Autodesk Fusion 360 part; units mm, degrees
sketch "Sketch1" plane through (0, 0, 0) normal (0, 0, 1) x (1, 0, 0)
  line L0 (-1.1, 1.1) -> (-1.1, 5.1)
  arc A0 (1.1, 5.1) -> (-1.1, 5.1) centre (0, 5.1) ccw
  line L1 (1.1, 5.1) -> (1.1, 1.1)
  line L2 (-1.1, 5.1) -> (1.1, 5.1) construction
  line L3 (1.1, 1.1) -> (-1.1, 1.1) construction
  line L4 (-1.1, 1.1) -> (-1.1, -1.1) construction
  line L5 (-1.1, -1.1) -> (1.1, -1.1) construction
  line L6 (1.1, -1.1) -> (1.1, 1.1) construction
  line L7 (1.1, 1.1) -> (-1.1, -1.1) construction
  line L8 (-1.1, 1.1) -> (1.1, -1.1) construction
  line L9 (-1.1, -1.1) -> (-5.1, -1.1)
  arc A1 (-5.1, 1.1) -> (-5.1, -1.1) centre (-5.1, 0) ccw
  line L10 (-5.1, 1.1) -> (-1.1, 1.1)
  line L11 (1.1, -1.1) -> (1.1, -5.1)
  arc A2 (-1.1, -5.1) -> (1.1, -5.1) centre (0, -5.1) ccw
  line L12 (-1.1, -5.1) -> (-1.1, -1.1)
  line L13 (1.1, 1.1) -> (5.1, 1.1)
  arc A3 (5.1, -1.1) -> (5.1, 1.1) centre (5.1, 0) ccw
  line L14 (5.1, -1.1) -> (1.1, -1.1)
  line L15 (7.1, 7.1) -> (-7.1, 7.1)
  line L16 (-7.1, 7.1) -> (-7.1, -7.1)
  line L17 (-7.1, -7.1) -> (7.1, -7.1)
  line L18 (7.1, -7.1) -> (7.1, 7.1)
  line L19 (7.1, 7.1) -> (-7.1, -7.1) construction
  line L20 (-7.1, 7.1) -> (7.1, -7.1) construction
  dimension "d2" = 2.2
  dimension "d3" = 2.2
  dimension "d4" = 2.2
  dimension "d5" = 4
  dimension "d7" = 360
  dimension "d37" = 2
extrude "Extrude1" add sketch "Sketch1" along normal blind 3
sketch "Sketch2" plane through (0, 0, 0) normal (0, 0, 1) x (1, 0, 0)
  line L0 (-33.9, 6.35) -> (-21.2, 6.35) construction
  line L1 (-21.2, 6.35) -> (-21.2, -6.35) construction
  line L2 (-21.2, -6.35) -> (-33.9, -6.35) construction
  line L3 (-33.9, -6.35) -> (-33.9, 6.35) construction
  line L4 (21.2, 6.35) -> (33.9, 6.35) construction
  line L5 (33.9, 6.35) -> (33.9, -6.35) construction
  line L6 (33.9, -6.35) -> (21.2, -6.35) construction
  line L7 (21.2, -6.35) -> (21.2, 6.35) construction
  line L8 (-21.2, 0) -> (21.2, 0) construction
  line L9 (-21.1, -6.45) -> (-34, -6.45)
  line L10 (-34, -6.45) -> (-34, 6.45)
  line L11 (-34, 6.45) -> (-21.1, 6.45)
  line L12 (-21.1, 6.45) -> (-21.1, -6.45)
  line L13 (-18.6, -8.95) -> (-36.5, -8.95)
  line L14 (-36.5, -8.95) -> (-36.5, 8.95)
  line L15 (-36.5, 8.95) -> (-18.6, 8.95)
  line L16 (-18.6, 8.95) -> (-18.6, -8.95)
  line L17 (0, 2.5) -> (0, 20)
  line L18 (34, -6.45) -> (34, 6.45)
  line L19 (34, 6.45) -> (21.1, 6.45)
  line L20 (21.1, 6.45) -> (21.1, -6.45)
  line L21 (21.1, -6.45) -> (34, -6.45)
  line L22 (36.5, -8.95) -> (36.5, 8.95)
  line L23 (36.5, 8.95) -> (18.6, 8.95)
  line L24 (18.6, -8.95) -> (36.5, -8.95)
  line L25 (18.6, 8.95) -> (18.6, -8.95)
  line L26 (-18.6, -2.6) -> (-18.6, -8.95)
  line L27 (-18.6, 8.95) -> (18.6, 8.95)
  line L28 (18.6, -8.95) -> (-18.6, -8.95)
  line L29 (-7.1, 7.1) -> (-7.1, -7.1)
  line L30 (-7.1, -7.1) -> (7.1, -7.1)
  line L31 (7.1, -7.1) -> (7.1, 7.1)
  line L32 (7.1, 7.1) -> (-7.1, 7.1)
  dimension "d18" = 12.7
  dimension "d19" = 12.7
  dimension "d20" = 42.4
  dimension "d23" = -2.5
extrude "Extrude2" add sketch "Sketch2" along normal blind 3
extrude "Extrude3" add sketch "Sketch2" against normal blind 19 contours L13 L14 L15 L16 L26 | L22 L23 L24 L25
fillet "Fillet1" radius 12 2 edges at (-18.6, 0, 0) (18.6, 0, 0)
sketch "Sketch3" plane through (0, 8.95, 0) normal (0, 1, 0) x (-1, 0, 0)
  line L0 (36.5, -19) -> (36.5, 3)
  line L1 (36.5, 3) -> (-36.5, 3)
  line L2 (18.6, -12) -> (18.6, -19)
  line L3 (-36.5, -19) -> (-18.6, -19)
  circle A0 centre (-27.55, -12.6) radius 2.075
  circle A1 centre (-27.55, -2.6) radius 2.075
  line L4 (-27.55, -19) -> (-27.55, 3) construction
  line L5 (-36.5, 3) -> (-36.5, -19)
  line L6 (-18.6, -19) -> (-18.6, -12)
  line L7 (18.6, -19) -> (36.5, -19)
  line L8 (0, 1.75) -> (0, 22.5)
  circle A2 centre (27.55, -12.6) radius 2.075
  circle A3 centre (27.55, -2.6) radius 2.075
  dimension "d32" = 4.15
  dimension "d33" = 10
  dimension "d34" = 5.6
extrude "Extrude4" cut sketch "Sketch3" against normal blind 17.9
sketch "Sketch4" plane through (0, 0, 3) normal (0, 0, 1) x (1, 0, 0)
  line L0 (36.5, -8.95) -> (36.5, 8.95)
  line L1 (36.5, 8.95) -> (-36.5, 8.95)
  line L2 (-36.5, 8.95) -> (-36.5, -8.95)
  line L3 (-36.5, -8.95) -> (36.5, -8.95)
  line L4 (-34, 6.45) -> (-21.1, 6.45)
  line L5 (-21.1, 6.45) -> (-21.1, -6.45)
  line L6 (-21.1, -6.45) -> (-34, -6.45)
  line L7 (-34, -6.45) -> (-34, 6.45)
  line L8 (34, -6.45) -> (21.1, -6.45)
  line L9 (21.1, -6.45) -> (21.1, 6.45)
  line L10 (21.1, 6.45) -> (34, 6.45)
  line L11 (34, 6.45) -> (34, -6.45)
  arc A0 (1.1, 5.1) -> (-1.1, 5.1) centre (0, 5.1) ccw
  line L12 (1.1, 5.1) -> (1.1, 1.1)
  line L13 (1.1, 1.1) -> (5.1, 1.1)
  arc A1 (5.1, -1.1) -> (5.1, 1.1) centre (5.1, 0) ccw
  line L14 (5.1, -1.1) -> (1.1, -1.1)
  line L15 (1.1, -1.1) -> (1.1, -5.1)
  arc A2 (-1.1, -5.1) -> (1.1, -5.1) centre (0, -5.1) ccw
  line L16 (-1.1, -5.1) -> (-1.1, -1.1)
  line L17 (-1.1, -1.1) -> (-5.1, -1.1)
  arc A3 (-5.1, 1.1) -> (-5.1, -1.1) centre (-5.1, 0) ccw
  line L18 (-5.1, 1.1) -> (-1.1, 1.1)
  line L19 (-1.1, 1.1) -> (-1.1, 5.1)
  line L20 (-21.1, 6.45) -> (-21.1, -6.45)
  line L21 (21.1, -6.45) -> (21.1, 6.45)
  line L22 (-21.1, 0) -> (21.1, 0) construction
  circle A4 centre (-14.1, 0) radius 2.075
  line L23 (0, 2.5) -> (0, 20)
  circle A5 centre (14.1, 0) radius 2.075
  dimension "d38" = 7
  dimension "d39" = 4.15
extrude "Extrude5" cut sketch "Sketch4" against normal blind 22 contours A4 | A5
ref_plane "WorkPlane1" through (0, 0, -6) normal (0, 0, -1) x (-1, 0, 0)
sketch "Sketch5" plane through (0, 0, -6) normal (0, 0, -1) x (-1, 0, 0)
  line L0 (-21.1, 6.45) -> (-21.1, -6.45)
  line L1 (21.1, -6.45) -> (21.1, 6.45)
  line L2 (-21.1, 0) -> (21.1, 0) construction
  circle A0 centre (-14.1, 0) radius 4.5
  line L3 (0, 1.75) -> (0, 22.5)
  circle A1 centre (14.1, 0) radius 4.5
  line L4 (-17.7, 2.7) -> (-17.7, -2.7)
  line L5 (17.7, 2.7) -> (17.7, -2.7)
  dimension "d43" = 9
  dimension "d44" = 7
  dimension "d49" = 3.6
extrude "Extrude6" cut sketch "Sketch5" along normal blind -6 and the other way blind -45.366 contours A0 L4 | A1 L5 picked at (-15.387, 1.0056) picked at (17.8896, 0.5649)
equation "mounting_size = 2.2 mm"
equation "d2 = mounting_size"
equation "d3 = mounting_size"
equation "d4 = mounting_size"
equation "tolerance_bar = 0.1 mm"
equation "d30 = 13 mm - ( 4 / 4 ) * 1 mm"
equation "tolerance_hole = 0.15 mm"
equation "d32 = 4 mm + tolerance_hole"
equation "d39 = 4 mm + tolerance_hole"
equation "d49 = ( 7 / 2 ) * 1 mm + 0.1 mm"
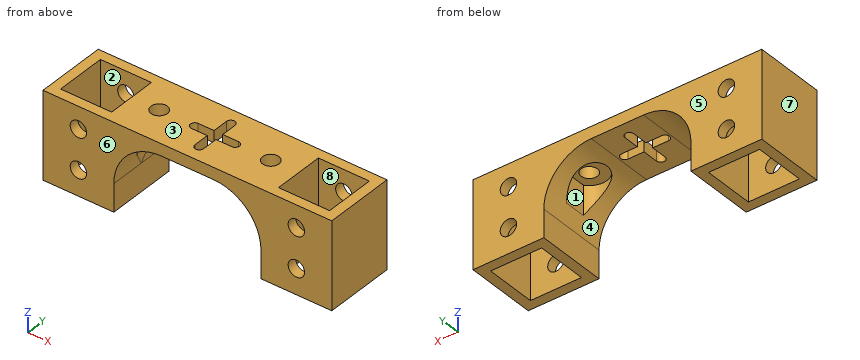
CAD build for the part. Positions are in the model's coordinates, mm. Face numbers are marked on the shaded views. A direction names the side the tool comes from. Round coordinates to 2 decimals unless told otherwise and drop trailing zeros. Write each loop counter-clockwise with the first axis right and the second up, starting at its lowest first coordinate (ties: lowest second). Pieces come first, ordered by that corner, then holes. Notation, with made-up numbers: (47, -29.5) - (71, -29.5) arc R17 ccw to (71, -9.5) - close; hole circle Ø3 at (85.25, 8). An arc over 180 degrees is marked (long way). Return JSON: item names as keys, results as strings. Group by question number.
Item 1: Band-saw the part on D-D on y = -7.5. List the corners of the cut face in (x, z) (3 decimals).
Item 2: 3-axis set-ups, long thin cutter, end or side, ignore diameter. For the marked faces 1, 2, 3, 4 and 5: which of +Z, -Z, +X, -X, +Y, -Y reach the whole face in a straight line?
Item 3: Band-saw the part on C-C on x = -27.55. List the corners of the cut face in (y, z) (3 decimals), plus the area to 3 significant figures.
Item 4: Band-saw the part on A-A on x = 3. List the corners of the cut face in (y, z).
Item 5: Band-saw the part on B-B on z = 1.5. List the corners of the cut face in (x, y) (3 decimals), plus the area to 3 significant figures.
Item 6: Probe probe 1 along X at (y, z) = (5.5, -13.25); probe 2 along X at (y, z) = (0, -4) (3 decimals); probe 3 along Y at (x, z) = (31.5, 0.5). List the from-to ranges inside material, lowest first.
Item 7: Flat gauge pins, fed straight in: pin 1 Ø0.7 at (x, y) = (-18, -0.5) entering from -Z; pin 2 Ø6.5 at (x, z) = (-27.55, -2.6) entering from -Y; pin 3 Ø3.5 at (x, z) = (27.55, -12.6) entering from -Y; pin 4 Ø10.5 at (x, y) = (-1, -4.5) entering from -Z. Where does each tip first touch, or does it go through?
Item 8: Mould opens along Y. For the marked faces 6, 7 and 8 say: +Y half, -Y half, draft (parallel to the pull), parting line (faces both ways), or undercut.
Resolved:
{
 "1": {"outline": "(-36.5, -19) - (-18.6, -19) - (-18.6, -12) arc R12 cw to (-6.6, 0) - (6.6, 0) arc R12 cw to (18.6, -12) - (18.6, -19) - (36.5, -19) - (36.5, 3) - (-36.5, 3) - close; hole circle Ø4.15 at (-27.55, -12.6); hole circle Ø4.15 at (-27.55, -2.6); hole circle Ø4.15 at (27.55, -12.6); hole circle Ø4.15 at (27.55, -2.6)"},
 "2": {"face 1": "-Z", "face 2": "+Z, -Z", "face 3": "+Z, +X, -X, +Y, -Y", "face 4": "-Z, +Y, -Y", "face 5": "+Z, -Z, +X, -X, +Y"},
 "3": {"outline": "(-8.95, -19) - (-6.45, -19) - (-6.45, -14.675) - (-8.95, -14.675) - close; (-8.95, -10.525) - (-6.45, -10.525) - (-6.45, -4.675) - (-8.95, -4.675) - close; (-8.95, -0.525) - (-6.45, -0.525) - (-6.45, 3) - (-8.95, 3) - close; (6.45, -19) - (8.95, -19) - (8.95, -14.675) - (6.45, -14.675) - close; (6.45, -10.525) - (8.95, -10.525) - (8.95, -4.675) - (6.45, -4.675) - close; (6.45, -0.525) - (8.95, -0.525) - (8.95, 3) - (6.45, 3) - close", "area": "68.5 mm²"},
 "4": {"outline": "(-8.95, 0) - (-1.1, 0) - (-1.1, 3) - (-8.95, 3) - close; (1.1, 0) - (8.95, 0) - (8.95, 3) - (1.1, 3) - close"},
 "5": {"outline": "(-36.5, -8.95) - (36.5, -8.95) - (36.5, 8.95) - (-36.5, 8.95) - close; hole (-34, -6.45) - (-21.1, -6.45) - (-21.1, 6.45) - (-34, 6.45) - close; hole circle Ø4.15 at (-14.1, 0); hole (-5.1, -1.1) - (-1.1, -1.1) - (-1.1, -5.1) arc R1.1 ccw to (1.1, -5.1) - (1.1, -1.1) - (5.1, -1.1) arc R1.1 ccw to (5.1, 1.1) - (1.1, 1.1) - (1.1, 5.1) arc R1.1 ccw to (-1.1, 5.1) - (-1.1, 1.1) - (-5.1, 1.1) arc R1.1 ccw to start; hole circle Ø4.15 at (14.1, 0); hole (21.1, -6.45) - (34, -6.45) - (34, 6.45) - (21.1, 6.45) - close", "area": "899 mm²"},
 "6": {"probe 1": "x = -36.5 to -34, -21.1 to -18.6, 18.6 to 21.1, 34 to 36.5", "probe 2": "x = -36.5 to -34, -21.1 to -18.6, -17.7 to -16.175, 17.7 to 21.1, 34 to 36.5", "probe 3": "y = -8.95 to -6.45, 6.45 to 8.95"},
 "7": {"pin 1": "stops at z = -7.44", "pin 2": "stops at y = -8.95", "pin 3": "passes through", "pin 4": "stops at z = 0"},
 "8": {"face 6": "-Y half", "face 7": "draft", "face 8": "undercut"}
}
